```python
from build123d import *

# Parameters (mm, degrees)
SKETCH1_W           = 152.4
SKETCH1_H           = 50.8
SKETCH1_R           = 1.5875
BOSS_EXTRUDE1_DEPTH = 19.05
SKETCH2_R           = 5.55625
CUT_EXTRUDE1_DEPTH  = 6.35


with BuildPart() as part:
    # Sketch1 → Boss-Extrude1 (new body)
    with BuildSketch(Plane(origin=(0, 0, 0), x_dir=(1, 0, 0), z_dir=(0, 1, 0))):
        with Locations((76.2, -25.4)):
            Rectangle(SKETCH1_W, SKETCH1_H)
        with Locations(Location((57.15, -12.7, 0), (0, 0, 270))):  # turned: the seam where the file's is
            Circle(SKETCH1_R, mode=Mode.SUBTRACT)
        with Locations(Location((57.15, -38.1, 0), (0, 0, 270))):  # turned: the seam where the file's is
            Circle(SKETCH1_R, mode=Mode.SUBTRACT)
        with Locations(Location((95.25, -12.7, 0), (0, 0, 270))):  # turned: the seam where the file's is
            Circle(SKETCH1_R, mode=Mode.SUBTRACT)
        with Locations(Location((95.25, -38.1, 0), (0, 0, 270))):  # turned: the seam where the file's is
            Circle(SKETCH1_R, mode=Mode.SUBTRACT)
        with Locations(Location((19.05, -15.875, 0), (0, 0, 270))):  # turned: the seam where the file's is
            Circle(SKETCH1_R, mode=Mode.SUBTRACT)
        with Locations(Location((19.05, -34.925, 0), (0, 0, 270))):  # turned: the seam where the file's is
            Circle(SKETCH1_R, mode=Mode.SUBTRACT)
        with Locations(Location((133.35, -15.875, 0), (0, 0, 270))):  # turned: the seam where the file's is
            Circle(SKETCH1_R, mode=Mode.SUBTRACT)
        with Locations(Location((133.35, -34.925, 0), (0, 0, 270))):  # turned: the seam where the file's is
            Circle(SKETCH1_R, mode=Mode.SUBTRACT)
    extrude(amount=BOSS_EXTRUDE1_DEPTH)

    # Sketch2 → Cut-Extrude1 (cut)
    with BuildSketch(Plane(origin=(0, 0, 0), x_dir=(-1, 0, 0), z_dir=(0, -1, 0))):
        with Locations(Location((-19.05, -34.925, 0), (0, 0, 90))):  # turned: the seam where the file's is
            Circle(SKETCH2_R)
        with Locations(Location((-19.05, -15.875, 0), (0, 0, 90))):  # turned: the seam where the file's is
            Circle(SKETCH2_R)
        with Locations(Location((-57.15, -38.1, 0), (0, 0, 90))):  # turned: the seam where the file's is
            Circle(SKETCH2_R)
        with Locations(Location((-57.15, -12.7, 0), (0, 0, 90))):  # turned: the seam where the file's is
            Circle(SKETCH2_R)
        with Locations(Location((-95.25, -38.1, 0), (0, 0, 90))):  # turned: the seam where the file's is
            Circle(SKETCH2_R)
        with Locations(Location((-95.25, -12.7, 0), (0, 0, 90))):  # turned: the seam where the file's is
            Circle(SKETCH2_R)
        with Locations(Location((-133.35, -15.875, 0), (0, 0, 90))):  # turned: the seam where the file's is
            Circle(SKETCH2_R)
        with Locations(Location((-133.35, -34.925, 0), (0, 0, 90))):  # turned: the seam where the file's is
            Circle(SKETCH2_R)
    extrude(amount=-CUT_EXTRUDE1_DEPTH, mode=Mode.SUBTRACT)


solid = part.part
```
The listing builds one solid part. Answer for the finished solid, in the listing's coordinates (mm). A direction names the side the tool comes from. Give positions to 0.01 mm unless a question says otherwise; leave off trailing zeros. Loops run counter-clockwise (first coordinate to the right, second up) from the corner with the lowest first, then second, coordinate; pieces in that order, holes last. Notation, with made-up numbers: M 21,18 L 57,18 A14 ccw 57,30 Z; hole C 34.25,20 d3. An arc over 180 degrees is marked long. One line per item, written item: value.
Q1. Flat-ended cylindrical pins translate along their axes: P1, Ø3, axis at x = 57.15, z = 12.7, coming from the -Y side; P2, Ø3.5, axis at x = 136, z = 14, coming from the -Y side. Find the tip coordinate at first contact, or state that the pin passes through.
Working result:
P1: passes through
P2: stops at y = 6.35
Q2. Determine the mould class of faces 3 (the face through (95.727, 12.611, 14.214)), 4 (the face through (75, 9, 50.8)), 5 (the face through (75, 9, 0)) for opening direction Z: +Z half, -Z half, draft (parallel to the pull), parting line (faces both ways), or undercut.
Working result:
face 3: undercut
face 4: +Z half
face 5: -Z half
Q3. For faces 1 (the face through (94.09, 6.35, 39.41)), 2 (the face through (134.924, 12.611, 15.668)), determine the directions among +Z, -Z, +X, -X, +Y, -Y from which every point of the face is accessible in a straight line to the end or side of a thin tool.
Working result:
face 1: -Y
face 2: +Y, -Y
Q4. Find the intervals of material crossed by line 1 (Z direction, x = 57.15, y = 16.75); line 2 (X direction, y = 10.25, z = 38.1); line 3 (Z direction, x = 133.35, y = 12.5), in increasing order. Write a range as from..to.
Working result:
line 1: z = 0..11.11, 14.29..36.51, 39.69..50.8
line 2: x = 0..55.56, 58.74..93.66, 96.84..152.4
line 3: z = 0..14.29, 17.46..33.34, 36.51..50.8
Q5. A cutting plane is placed at A-A on x = 133.35. Determine the outline of the cut face in (y, z).
Working result:
outline: M 0,0 L 19.05,0 L 19.05,14.29 L 6.35,14.29 L 6.35,10.32 L 0,10.32 Z; M 0,21.43 L 6.35,21.43 L 6.35,17.46 L 19.05,17.46 L 19.05,33.34 L 6.35,33.34 L 6.35,29.37 L 0,29.37 Z; M 0,40.48 L 6.35,40.48 L 6.35,36.51 L 19.05,36.51 L 19.05,50.8 L 0,50.8 Z
Q6. A cutting plane is placed at B-B on z = 12.5. Determine the outline of the cut face in (x, y), then the cut area to 3 significant figures.
Working result:
outline: M 0,0 L 14.64,0 L 14.64,6.35 L 23.46,6.35 L 23.46,0 L 51.6,0 L 51.6,6.35 L 55.58,6.35 L 55.58,19.05 L 0,19.05 Z; M 58.72,6.35 L 62.7,6.35 L 62.7,0 L 89.7,0 L 89.7,6.35 L 93.68,6.35 L 93.68,19.05 L 58.72,19.05 Z; M 96.82,6.35 L 100.8,6.35 L 100.8,0 L 128.94,0 L 128.94,6.35 L 137.76,6.35 L 137.76,0 L 152.4,0 L 152.4,19.05 L 96.82,19.05 Z
area: 2,570 mm^2
Q7. A cutting plane is placed at C-C on z = 38.1. Determine the outline of the cut face in (x, y), then the cut area to 3 significant figures.
Working result:
outline: M 0,0 L 14.49,0 L 14.49,6.35 L 23.61,6.35 L 23.61,0 L 51.59,0 L 51.59,6.35 L 55.56,6.35 L 55.56,19.05 L 0,19.05 Z; M 58.74,6.35 L 62.71,6.35 L 62.71,0 L 89.69,0 L 89.69,6.35 L 93.66,6.35 L 93.66,19.05 L 58.74,19.05 Z; M 96.84,6.35 L 100.81,6.35 L 100.81,0 L 128.79,0 L 128.79,6.35 L 137.91,6.35 L 137.91,0 L 152.4,0 L 152.4,19.05 L 96.84,19.05 Z
area: 2,570 mm^2
